```python
from build123d import *

# Parameters (mm, degrees)
F0_W     = 60.0074976683
F0_H     = 69.5122331381
F1_DEPTH = 50.8
F3_DEPTH = 50.8
F5_DEPTH = 25.4
F6_R     = 13.6924053839
F7_DEPTH = 25.4
F8_R     = 5.2161873837
F9_DEPTH = 50.8


with BuildPart() as f1:
    # F0 (on Front) → F1 (new body)
    with BuildSketch(Plane.XZ):
        with Locations((30.0037488341, 34.756116569)):
            Rectangle(F0_W, F0_H)
    extrude(amount=F1_DEPTH)

    # F2 (on face) → F3 (cut)
    with BuildSketch(Plane.XZ.offset(50.8)):
        with BuildLine():
            Line((60.0074976683, 69.5122331381), (41.8492034078, 69.5122331381))
            add(Edge.make_bspline(
                [(41.8492034078, 69.5122331381), (40.5229985665, 50.963393388), (38.2921086092, 19.7612600302), (53.7421113163, 9.5369669805), (60.0074976683, 5.3907446563)],
                knots=[0, 0, 0, 0, 0.5944734463, 1, 1, 1, 1], degree=3))
            Line((60.0074976683, 5.3907446563), (60.0074976683, 69.5122331381))
        make_face()
        with BuildLine():
            add(Edge.make_bspline(
                [(16.3140948862, 69.5122331381), (19.1757238105, 52.1069225067), (24.1823454085, 21.6551041788), (7.2530413082, 9.4744311002), (0, 4.255851265)],
                knots=[0, 0, 0, 0, 0.571568845, 1, 1, 1, 1], degree=3))
            Line((16.3140948862, 69.5122331381), (0, 69.5122331381))
            Line((0, 69.5122331381), (0, 4.255851265))
        make_face()
    extrude(amount=-F3_DEPTH, mode=Mode.SUBTRACT)

    # F4 (on face) → F5 (cut)
    with BuildSketch(Plane.XZ.offset(50.8)):
        with BuildLine():
            add(Edge.make_bspline(
                [(16.3140948862, 69.5122331381), (19.1757238105, 52.1069225067), (24.1823454085, 21.6551041788), (7.2530413082, 9.4744311002), (0, 4.255851265)],
                knots=[0, 0, 0, 0, 0.571568845, 1, 1, 1, 1], degree=3))
            Line((0, 4.255851265), (60.0074976683, 4.255851265))
            Line((60.0074976683, 4.255851265), (60.0074976683, 5.3907446563))
            add(Edge.make_bspline(
                [(41.8492034078, 69.5122331381), (40.5229985665, 50.963393388), (38.2921086092, 19.7612600302), (53.7421113163, 9.5369669805), (60.0074976683, 5.3907446563)],
                knots=[0, 0, 0, 0, 0.5944734463, 1, 1, 1, 1], degree=3))
            Line((41.8492034078, 69.5122331381), (16.3140948862, 69.5122331381))
        make_face()
    extrude(amount=-F5_DEPTH, mode=Mode.SUBTRACT)

    # F6 (on face) → F7 (join)
    with BuildSketch(Plane.XZ.offset(25.4)):
        with Locations((28.5142045468, 61.5679770708)):
            Circle(F6_R)
    extrude(amount=F7_DEPTH)

    # F8 (on face) → F9 (cut)
    with BuildSketch(Plane.XZ.offset(50.8)):
        with Locations((27.9467590153, 63.8377666473)):
            Circle(F8_R)
    extrude(amount=-F9_DEPTH, mode=Mode.SUBTRACT)


solid = f1.part
```
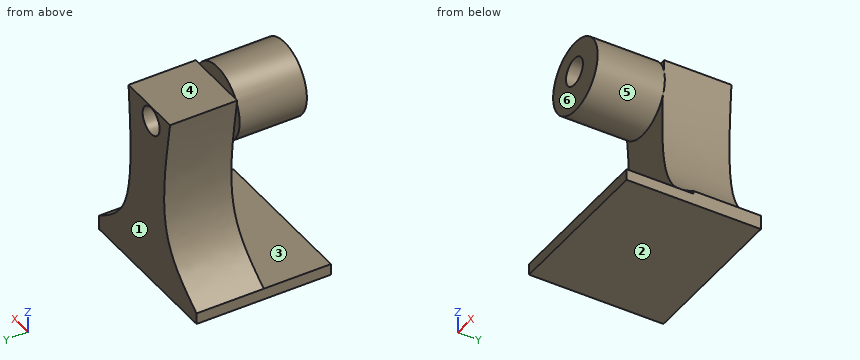
Geometry check sheet. Reference: the model listing, model coordinates, mm. Face numbers are marked on the shaded views. A direction names the side the tool comes from. Coordinates: 2 decimals unless noted, no trailing zeros. Write each loop counter-clockwise with the first axis right and the second up, starting at its lowest first coordinate (ties: lowest second). Pieces come first, ordered by that corner, then holes. Notation, with made-up numbers: M 84.5,62 L 94.5,62 A24 cw 94.5,95 Z; hole C 40,34 d8. An arc over 180 degrees is marked long. Use one line per item in the form item = value. Start each with the question number.
1) Section check A-A on y = -40.5. Enter the section's corners in (x, z).
2) Go/stop test with flat-tipped pins: pin 1 Ø4 at (y, z) = (-20.5, 41.5) entering from +X; pin 2 Ø1.5 at (y, z) = (-9, 56.5) entering from -X; pin 3 Ø3 at (x, z) = (24.5, 13) entering from -Y; pin 4 Ø8 at (x, z) = (48, 40) entering from -Y. Record where each tip stops, or that it passes through.
3) Release check for a two-part mould opening along Z. For the marked faces 1, 2 and 3 record: pulls with the +Z half, pulls with the -Z half, needs draft (parallel to the pull), parting line crosses it, or undercut.
4) Section check B-B on x = 25. Enter the section's corners in (y, z).
5) Section check C-C on x = 35. Enter the section's corners in (y, z).
6) Thickness scan on probe 1 along Z at (x, y) = (6, -26.5); probe 2 along Y at (x, z) = (19.5, 70); probe 3 along Z at (x, y) = (20, -37). Record the ranges inside material, lowest first. Write a range as from..to.
7) Set-up check for the marked faces 4, 5 and 6: record each of +Z, -Z, +X, -X, +Y, -Y from which the full face is reachable in a straight line by a thin tool's end or side.
Responses:
q1.outline = M 0,0 L 60.01,0 L 60.01,4.26 L 0,4.26 Z; C 28.51,61.57 d27.38; hole C 27.95,63.84 d10.43
q2.pin_1 = 40.72
q2.pin_2 = 18.25
q2.pin_3 = -25.4
q2.pin_4 = through
q3.face_1 = needs draft
q3.face_2 = pulls with the -Z half
q3.face_3 = undercut
q4.outline = M -50.8,0 L 0,0 L 0,59.53 L -50.8,59.53 L -50.8,48.33 L -25.4,48.33 L -25.4,4.26 L -50.8,4.26 Z; M -50.8,68.14 L 0,68.14 L 0,69.51 L -25.4,69.51 L -25.4,74.8 L -50.8,74.8 Z
q5.outline = M -50.8,0 L 0,0 L 0,69.51 L -25.4,69.51 L -25.4,73.63 L -50.8,73.63 L -50.8,49.51 L -25.4,49.51 L -25.4,4.26 L -50.8,4.26 Z
q6.probe_1 = 0..4.26
q6.probe_2 = -50.8..-25.4
q6.probe_3 = 0..4.26, 50.84..72.29
q7.face_4 = +Z, +X, -X, +Y
q7.face_5 = -Y
q7.face_6 = +Z, -Z, +X, -X, -Y
